Source: CAD feature listing. Evaluate the final solid. Frame: model axes, mm. Face numbers are marked on the shaded views. A direction names the side the tool comes from. Round coordinates to 2 decimals unless told otherwise and drop trailing zeros. Write each loop counter-clockwise with the first axis right and the second up, starting at its lowest first coordinate (ties: lowest second). Pieces come first, ordered by that corner, then holes. Notation, with made-up numbers: M -19,76.5 L 34,76.5 A17 ccw 34,81.5 Z; hole C -8.75,-4 d6. An arc over 180 degrees is marked long. Answer in a Markdown table with one row per item. Add a question column.
Item 1: Mould query, pull axis X, two halves, no side actions, for the marked faces 1, 2, 3 and 4. Classes: released by +X, released by -X, zero draft, split by the parting line, or undercut.
Item 2: Cut plane B-B on z = 26.75. Return loops of the section in (x, y), and give its area (3 significant figures).
Item 3: Material intervals for probe 1 along Z at (x, y) = (-55.25, 62.75); probe 2 along X at (y, z) = (64.75, 21.5); probe 3 along Y at (x, z) = (-64, 25), sorted ascending.
Item 4: Cut plane C-C on z = 19.75. Return loops of the section in (x, y).
Item 5: Cut plane A-A on z = 15.25. Return loops of the section in (x, y).
Item 6: Cut plane D-D on x = -69.25. Return loops of the section in (y, z), and give its area (3 significant figures).
Item 7: Set-up query: the marked faces 5, 6, 7 and 8. Return all of +Z, -Z, +X, -X, +Y, -Y with unobstructed straight access to the full face (end or side cutting, diameter ignored); none if empty.
Item 8: Contact query for flat-ended pins moving along their axis: pin 1 (1.6 mm diameter, centred on x = -50, y = 66.5, fed in from -Z); pin 2 (5 mm diameter, centred on x = -58, z = 9, fed in from +Y); pin 3 (3 mm diameter, centred on y = 49.5, z = 15, fed in from -X). Output: stop coordinate, or through.
from build123d import *

# Parameters (mm, degrees)
SKETCH077_W             = 30
SKETCH077_H             = 6
PAD034_DEPTH            = 28
SKETCH078_R             = 11.25
POCKET039_DEPTH         = 3
SKETCH079_R             = 1.2
POCKET040_DEPTH         = 3
SKETCH080_R             = 1.65
POCKET041_DEPTH         = 7
SKETCH081_R             = 1.65
POCKET042_DEPTH         = 8
BODY024_PLACEMENT_ANGLE = 225


with BuildPart() as part:
    # Sketch077 → Pad034 (new body)
    with BuildSketch(Plane.XY):
        Rectangle(SKETCH077_W, SKETCH077_H)
    extrude(amount=PAD034_DEPTH)

    # Sketch078 (on Face4 of Pad034) → Pocket039 (cut)
    with BuildSketch(Plane(origin=(0, 3, 0), x_dir=(-1, 0, 0), z_dir=(0, 1, 0))):
        with Locations((0, 15)):
            Circle(SKETCH078_R)
    extrude(amount=-POCKET039_DEPTH, mode=Mode.SUBTRACT)

    # Sketch079 (on Face8 of Pocket039) → Pocket040 (cut)
    with BuildSketch(Plane(origin=(0, 0, 0), x_dir=(-1, 0, 0), z_dir=(0, 1, 0))):
        with Locations((6.363961, 8.636039)):
            Circle(SKETCH079_R)
        with Locations((6.363961, 21.363961)):
            Circle(SKETCH079_R)
        with Locations((-6.363961, 21.363961)):
            Circle(SKETCH079_R)
        with Locations((-6.363961, 8.636039)):
            Circle(SKETCH079_R)
        with BuildLine():
            Line((-6.25, 18.674235), (-6.25, 11.325765))
            ThreePointArc((-6.25, 11.325765), (0, 7.75), (6.25, 11.325765))
            Line((6.25, 18.674235), (6.25, 11.325765))
            ThreePointArc((6.25, 18.674235), (0, 22.25), (-6.25, 18.674235))
        make_face()
    extrude(amount=-POCKET040_DEPTH, mode=Mode.SUBTRACT)

    # Sketch080 (on Face5 of Pocket040) → Pocket041 (cut)
    with BuildSketch(Plane.XY.offset(28)):
        with Locations((-12, 0)):
            Circle(SKETCH080_R)
        with Locations((12, 0)):
            Circle(SKETCH080_R)
    extrude(amount=-POCKET041_DEPTH, mode=Mode.SUBTRACT)

    # Sketch081 (on Face4 of Pocket041) → Pocket042 (cut)
    with BuildSketch(Plane(origin=(0, 0, 0), x_dir=(1, 0, 0), z_dir=(0, 0, -1))):
        with Locations((-12, 0)):
            Circle(SKETCH081_R)
        with Locations((12, 0)):
            Circle(SKETCH081_R)
    extrude(amount=-POCKET042_DEPTH, mode=Mode.SUBTRACT)


with BuildPart() as part_1:
    # Body024 placement: moved
    add(part.part.moved(Location((-58.5, 58.5, 2))).rotate(Axis((-58.5, 58.5, 2), (0, 0, 1)), BODY024_PLACEMENT_ANGLE))


solid = part_1.part
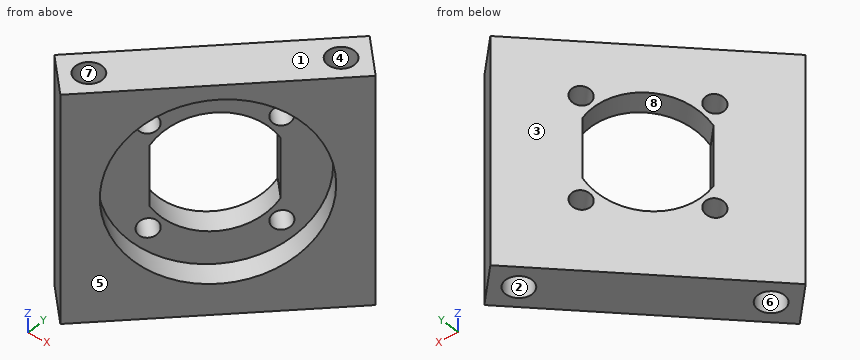
Results below:
| question | item | result |
|---|---|---|
| 1 | face 1 | zero draft |
| 1 | face 2 | undercut |
| 1 | face 3 | released by -X |
| 1 | face 4 | undercut |
| 2 | outline | M -71.23,50.01 L -66.99,45.77 L -60.35,52.41 L -62.47,54.53 L -54.53,62.47 L -52.41,60.35 L -45.77,66.99 L -50.01,71.23 Z; hole C -66.99,50.01 d3.3; hole C -50.01,66.99 d3.3 |
| 2 | area | 129 mm2 |
| 3 | probe 1 | 2 to 10.07, 11.2 to 12.06, 21.94 to 22.8, 23.93 to 30 |
| 3 | probe 2 | -56.49 to -52.25, -50.17 to -48.01 |
| 3 | probe 3 | 48.76 to 52.81, 53 to 57.24 |
| 4 | outline | M -71.23,50.01 L -66.99,45.77 L -64.09,48.67 L -66.21,50.79 L -62.92,54.08 L -65.04,56.2 Z; M -56.2,65.04 L -54.08,62.92 L -50.79,66.21 L -48.67,64.09 L -45.77,66.99 L -50.01,71.23 Z |
| 5 | outline | M -71.23,50.01 L -66.99,45.77 L -64.24,48.52 L -66.36,50.64 L -62.92,54.08 L -65.04,56.2 Z; M -56.2,65.04 L -54.08,62.92 L -50.64,66.36 L -48.52,64.24 L -45.77,66.99 L -50.01,71.23 Z |
| 6 | outline | M 48.04,2 L 51.99,2 L 51.99,30 L 48.04,30 Z |
| 6 | area | 111 mm2 |
| 7 | face 5 | +Z, -Z, +X, -Y |
| 7 | face 6 | -Z |
| 7 | face 7 | +Z |
| 7 | face 8 | none |
| 8 | pin 1 | z = 10 |
| 8 | pin 2 | y = 65.74 |
| 8 | pin 3 | x = -71.23 |
